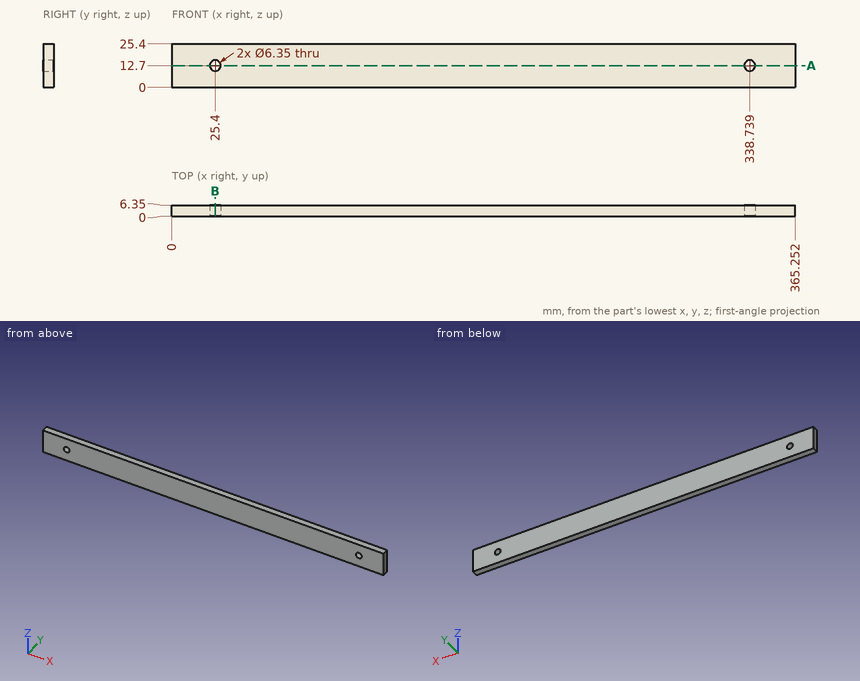
The drawing under review shows one solid part. Ordinate dimensions are in mm from its lowest x, y, z. Give positions to 0.01 mm unless a question says otherwise; leave off trailing zeros. Order: outer loops, then holes, each group sorted by start corner. A loop starts at its lowest first (then second) coordinate and runs counter-clockwise, first axis right, second up. Notation, with made-up numbers: M 69.5,61.25 L 74.5,61.25 A25 cw 74.5,75.25 Z; hole C 40.25,-35 d2. An arc over 180 degrees is marked long. Answer in a Markdown table with one row per item. Add a question column.
1. Add section B-B on x = 25.4. State the section outline as (y, z) points (3 decimals).
2. To check wall thickness, follow line 1 along X through (y, z) = (3, 12.7) (3 decimals); line 2 along X through (y, z) = (0.75, 13.75); line 3 along Z through (x, y) = (28, 3.25). State the ranges of each line that lie inside material, in increasing order.
3. Add section A-A on z = 12.7. State the section outline as (x, y) points (3 decimals).
The answers:
| question | item | result |
|---|---|---|
| 1 | outline | M 0,0 L 6.35,0 L 6.35,9.525 L 0,9.525 Z; M 0,15.875 L 6.35,15.875 L 6.35,25.4 L 0,25.4 Z |
| 2 | line 1 | 0 to 22.225, 28.575 to 335.564, 341.914 to 365.252 |
| 2 | line 2 | 0 to 22.4, 28.4 to 335.74, 341.74 to 365.25 |
| 2 | line 3 | 0 to 10.88, 14.52 to 25.4 |
| 3 | outline | M 0,0 L 22.225,0 L 22.225,6.35 L 0,6.35 Z; M 28.575,0 L 335.564,0 L 335.564,6.35 L 28.575,6.35 Z; M 341.914,0 L 365.252,0 L 365.252,6.35 L 341.914,6.35 Z |
